from build123d import *

# Parameters (mm, degrees)
SKETCH_2_R          = 2.5
CUT_EXTRUDE_2_DEPTH = 10
CHAMFER_1_SIZE      = 2
SCALE_1_SCALE       = 0.8
SCALE_2_SCALE       = 0.8
SCALE_3_SCALE       = 0.8


with BuildPart() as part:
    # 草图1 → 旋转1 (revolve)
    with BuildSketch(Plane.XY, mode=Mode.PRIVATE) as revolve_1_sk:
        Polygon((-10, 2), (-27, 2), (-27, 6), (-10, 6), (-10, 19), (-8, 19), (-8, 26), (-5, 26), (-5, 0), (-10, 0), align=None)
    revolve(revolve_1_sk.sketch.rotate(Axis((0, 0, 0), (0, -1, 0)), 270), axis=Axis((0, 0, 0), (0, -1, 0)))

    # 草图2 → 切除-拉伸2 (cut)
    with BuildSketch(Plane.XZ.offset(-2)):
        with Locations(Location((0, 22.5, 0), (0, 0, 270))):
            Circle(SKETCH_2_R)
        with Locations(Location((19.485571585, 11.25, 0), (0, 0, 270))):
            Circle(SKETCH_2_R)
        with Locations(Location((19.485571585, -11.25, 0), (0, 0, 270))):
            Circle(SKETCH_2_R)
        with Locations(Location((0, -22.5, 0), (0, 0, 270))):
            Circle(SKETCH_2_R)
        with Locations(Location((-19.485571585, -11.25, 0), (0, 0, 270))):
            Circle(SKETCH_2_R)
        with Locations(Location((-19.485571585, 11.25, 0), (0, 0, 270))):
            Circle(SKETCH_2_R)
    extrude(amount=-CUT_EXTRUDE_2_DEPTH, mode=Mode.SUBTRACT)

    # 倒角1
    chamfer_1_edges = [part.edges().sort_by_distance(p)[0] for p in [
        (0, 6, -10),
    ]]
    chamfer(chamfer_1_edges, length=CHAMFER_1_SIZE)


with BuildPart() as part_1:
    # 缩放比例1: scaled about (0, 0, 0)
    add(part.part.scale(SCALE_1_SCALE))


with BuildPart() as part_2:
    # 缩放比例2: scaled about (0, 0, 0)
    add(part_1.part.scale(SCALE_2_SCALE))


with BuildPart() as part_3:
    # 缩放比例3: scaled about (0, 0, 0)
    add(part_2.part.scale(SCALE_3_SCALE))


solid = part_3.part
The model under review builds one solid part; all positions refer to its coordinate system, in mm. A direction names the side the tool comes from. Coordinates: 2 decimals unless noted, no trailing zeros. Write each loop counter-clockwise with the first axis right and the second up, starting at its lowest first coordinate (ties: lowest second). Pieces come first, ordered by that corner, then holes. Notation, with made-up numbers: M -19.5,74 L 34.5,74 A13 cw 34.5,91 Z; hole C 11.25,7.25 d8. An arc over 180 degrees is marked long. Put each result on its own line as item: value.
1) Add section B-B on x = 0. State how many separate pieces and enclosed holes the cut face has, then the cut area to 3 significant figures.
Computed:
separate pieces: 4
enclosed holes: 0
area: 87.0 mm2
2) Add section C-C on x = -10.5. Give the boundary of the cut face in (y, z), then the cut area to 3 significant figures.
Computed:
outline: M 1.02,-8.99 L 3.07,-8.99 L 3.07,-6.93 L 1.02,-6.93 Z; M 1.02,-4.59 L 3.07,-4.59 L 3.07,4.59 L 1.02,4.59 Z; M 1.02,6.93 L 3.07,6.93 L 3.07,8.99 L 1.02,8.99 Z
area: 27.3 mm2
3) Clearance check with flat-ended pins moving along their axes: pin 1 Ø4 at (x, z) = (-3, -8) entering from -Y; pin 2 Ø6 at (x, y) = (5.5, 7) entering from -Z; pin 3 Ø1.5 at (y, z) = (12, -6.5) entering from +X; pin 4 Ø3.5 at (x, z) = (9.98, 5.76) entering from +Y. State where each tip first meets the part, or that it passes through.
Computed:
pin 1: stops at y = 1.02
pin 2: stops at z = -4.47
pin 3: passes through
pin 4: stops at y = 3.07
4) Add section A-A on z = 0. Give the boundary of the cut face in (x, y), then the cut area to 3 significant figures.
Computed:
outline: M -13.82,1.02 L -5.12,1.02 L -5.12,0 L -2.56,0 L -2.56,13.31 L -4.1,13.31 L -4.1,9.73 L -5.12,9.73 L -5.12,4.1 L -6.14,3.07 L -13.82,3.07 Z; M 2.56,0 L 5.12,0 L 5.12,1.02 L 13.82,1.02 L 13.82,3.07 L 6.14,3.07 L 5.12,4.1 L 5.12,9.73 L 4.1,9.73 L 4.1,13.31 L 2.56,13.31 Z
area: 97.5 mm2
5) Wall thickness on probe 1 along Y at (x, z) = (-4.75, -9); probe 2 along Z at (x, y) = (-1, 11.25); probe 3 along X at (y, z) = (1.9, -5.76): over which ranges is each line inside the solid? List them lowest first. Write a range as [from, to].
Computed:
probe 1: y = [1.02, 3.07]
probe 2: z = [-3.97, -2.36], [2.36, 3.97]
probe 3: x = [-12.57, -11.26], [-8.7, 8.7], [11.26, 12.57]
6) For faces 1 (the flat face through (-2, 13.312, 2)), 2 (the cylindrical face through (-1.538, 0.519, 4.884)), 3 (the cylindrical face through (-1.538, 6.951, 4.884)), list the 3-axis set-ups (+Z, -Z, +X, -X, +Y, -Y) from which the entire face can be reached by the end or side of a thin tool; tool diameter is ignored.
Computed:
face 1: +Z, -Z, +X, -X, +Y
face 2: -Y
face 3: +Y
7) Add section D-D on y = 2.25. Give the boundary of the cut face in (x, z), then the cut area to 3 significant figures.
Computed:
outline: C 0,0 d27.65; hole C -9.98,-5.76 d2.56; hole C -9.98,5.76 d2.56; hole C 0,0 d5.12; hole C 0,-11.52 d2.56; hole C 0,11.52 d2.56; hole C 9.98,-5.76 d2.56; hole C 9.98,5.76 d2.56
area: 549 mm2
